from build123d import *

# Parameters (mm, degrees)
BOSS_EXTRUDE1_DEPTH                            = 76.2
CUT_EXTRUDE1_DEPTH                             = 15.24
CUT_EXTRUDE2_DEPTH                             = 15.24
CSK_FOR_M3_FLAT_HEAD_MACHINE_SCREW1_AT_2_COUNT = 2
CSK_FOR_M3_FLAT_HEAD_MACHINE_SCREW1_AT_2_PITCH = 59.436
CSK_FOR_M3_FLAT_HEAD_MACHINE_SCREW1_AT_3_COUNT = 2
CSK_FOR_M3_FLAT_HEAD_MACHINE_SCREW1_AT_3_PITCH = 29.851441177
M3_5_CLEARANCE_HOLE1_D                         = 3.96875
M3_5_CLEARANCE_HOLE1_DEPTH                     = 15.24
M3_5_CLEARANCE_HOLE2_D                         = 3.96875
M3_5_CLEARANCE_HOLE2_DEPTH                     = 15.24
M3_5_CLEARANCE_HOLE3_D                         = 3.96875
M3_5_CLEARANCE_HOLE3_DEPTH                     = 45.72
SKETCH21_R                                     = 2.5
CUT_EXTRUDE3_DEPTH                             = 1.5748


with BuildPart() as part:
    # Sketch1 → Boss-Extrude1 (new body)
    with BuildSketch(Plane.XY.offset(38.1)):
        with BuildLine():
            Line((25.4, -2.950829012), (25.4, -1.376029012))
            Line((25.4, -1.376029012), (3.278975474, -1.376029012))
            ThreePointArc((3.278975474, -1.376029012), (-2.746946179, 2.258190135), (1.984375, -2.950829012))
            Line((1.984375, -2.950829012), (25.4, -2.950829012))
        make_face()
    extrude(amount=-BOSS_EXTRUDE1_DEPTH)

    # Sketch6 → Cut-Extrude1 (cut)
    with BuildSketch(Plane(origin=(0, 0, -22.86), x_dir=(-1, 0, 0), z_dir=(0, 0, -1))):
        with BuildLine():
            Line((-3.937, -1.376029012), (-3.937, -2.950829012))
            Line((-3.937, -2.950829012), (-1.984375, -2.950829012))
            ThreePointArc((-1.984375, -2.950829012), (2.746946179, 2.258190135), (-3.278975474, -1.376029012))
            Line((-3.278975474, -1.376029012), (-3.937, -1.376029012))
        make_face()
    extrude(amount=-CUT_EXTRUDE1_DEPTH, mode=Mode.SUBTRACT)

    # Sketch12 → Cut-Extrude2 (cut)
    with BuildSketch(Plane(origin=(0, 0, 7.62), x_dir=(-1, 0, 0), z_dir=(0, 0, -1))):
        with BuildLine():
            Line((-3.937, -1.376029012), (-3.937, -2.950829012))
            Line((-3.937, -2.950829012), (-1.984375, -2.950829012))
            ThreePointArc((-1.984375, -2.950829012), (2.746946179, 2.258190135), (-3.278975474, -1.376029012))
            Line((-3.278975474, -1.376029012), (-3.937, -1.376029012))
        make_face()
    extrude(amount=-CUT_EXTRUDE2_DEPTH, mode=Mode.SUBTRACT)

    # Sketch13 → CSK for M3 Flat Head Machine Screw1 (revolve, cut)
    with BuildSketch(Plane(origin=(16.637, -1.376029012, -29.718), x_dir=(0, 0, 1), z_dir=(1, 0, 0))):
        Polygon((0, 0), (0, 2.179970988), (1.7526, 2.179970988), (1.7526, 0.7874), (2.437076377, 0), align=None)
    csk_for_m3_flat_head_machine_screw1 = revolve(axis=Axis((16.637, 4.973970988, -29.718), (0, -1, 0)), mode=Mode.SUBTRACT)

    # CSK for M3 Flat Head Machine Screw1 at 2: CSK for M3 Flat Head Machine Screw1 ×2
    with Locations(*[(0, 0, i * CSK_FOR_M3_FLAT_HEAD_MACHINE_SCREW1_AT_2_PITCH) for i in range(1, CSK_FOR_M3_FLAT_HEAD_MACHINE_SCREW1_AT_2_COUNT)]):
        add(csk_for_m3_flat_head_machine_screw1, mode=Mode.SUBTRACT)

    # CSK for M3 Flat Head Machine Screw1 at 3: CSK for M3 Flat Head Machine Screw1 ×2
    with Locations(*[Vector(0.094447701, 0, 0.995529825) * (i * CSK_FOR_M3_FLAT_HEAD_MACHINE_SCREW1_AT_3_PITCH) for i in range(1, CSK_FOR_M3_FLAT_HEAD_MACHINE_SCREW1_AT_3_COUNT)]):
        add(csk_for_m3_flat_head_machine_screw1, mode=Mode.SUBTRACT)

    # M3.5 Clearance Hole1
    with Locations(Plane.XY.offset(38.1)):
        with Locations((0, 0)):
            Hole(M3_5_CLEARANCE_HOLE1_D / 2, depth=M3_5_CLEARANCE_HOLE1_DEPTH)

    # M3.5 Clearance Hole2
    with Locations(Plane(origin=(0, 0, -38.1), x_dir=(-1, 0, 0), z_dir=(0, 0, -1))):
        with Locations((0, 0)):
            Hole(M3_5_CLEARANCE_HOLE2_D / 2, depth=M3_5_CLEARANCE_HOLE2_DEPTH)

    # M3.5 Clearance Hole3
    with Locations(Plane(origin=(0, 0, -7.62), x_dir=(-1, 0, 0), z_dir=(0, 0, -1))):
        with Locations((0, 0)):
            Hole(M3_5_CLEARANCE_HOLE3_D / 2, depth=M3_5_CLEARANCE_HOLE3_DEPTH)

    # Sketch21 → Cut-Extrude3 (cut)
    with BuildSketch(Plane(origin=(0, -1.376029012, 0), x_dir=(1, 0, 0), z_dir=(0, 1, 0))):
        with Locations((16.637, 29.718)):
            Circle(SKETCH21_R)
        with Locations((19.4564, 0)):
            Circle(SKETCH21_R)
        with Locations((16.637, -29.718)):
            Circle(SKETCH21_R)
    extrude(amount=-CUT_EXTRUDE3_DEPTH, mode=Mode.SUBTRACT)


solid = part.part
Source: CAD feature listing. Evaluate the final solid. Frame: model axes, mm. A direction names the side the tool comes from. Coordinates: 2 decimals unless noted, no trailing zeros. Loops run counter-clockwise (first coordinate to the right, second up) from the corner with the lowest first, then second, coordinate; pieces in that order, holes last. Notation, with made-up numbers: (4, 54.25) - (51, 54.25) arc R30 ccw to (51, 92.25) - close; hole circle Ø3 at (5, 65). An arc over 180 degrees is marked (long way). One line per item, written item: value. Start each with the question number.
1. Ray query, L1, parallel to Z at x = 1.75, y = 1; L2, parallel to Y at x = 0, z = 31.75; L3, parallel to Z at x = 18.5, y = -2.25. Return the intervals inside material, ascending.
2. Contact query for flat-ended pins moving along their axis: P1, Ø1.3, axis at y = -2, z = -19, coming from the -X side; P2, Ø3, axis at x = 17, z = 22.5, coming from the +Y side; P3, Ø11.5, axis at x = 14.5, z = 3, coming from the -Y side. Output: stop coordinate, or through.
3. Section A-A (z = 0). Return the cut outline in (x, y).
4. Set-up query: faces 1 (the flat face through (3.937, -2, -15)), 2 (the cylindrical face through (14.65, -2.15, -28.2)). Return all of +Z, -Z, +X, -X, +Y, -Y with unobstructed straight access to the full face (end or side cutting, diameter ignored); none if empty.
5. Section B-B (x = 0). Return the cut outline in (y, z), and give its area (3 significant figures).
6. Section D-D (x = 15). Return the cut outline in (y, z).
7. Mould query, pull axis X, two halves, no side actions, for faces 3 (the flat face through (25.4, -2, 1)), 4 (the cylindrical face through (14.653, -2.152, 31.239)), 5 (the flat face through (14, -2.951, 1)). Classes: pulls with the +X half, pulls with the -X half, needs draft (parallel to the pull), parting line crosses it, or undercut.
Verdict:
1. L1: z = -38.1 to -22.86, -7.62 to 7.62, 22.86 to 38.1
1. L2: y = -3.56 to -1.98, 1.98 to 3.56
1. L3: z = -38.1 to -31.39, -28.05 to -2.31, 2.31 to 28.05, 31.39 to 38.1
2. P1: stops at x = 3.94
2. P2: stops at y = -1.38
2. P3: stops at y = -2.95
3. outline: (1.98, -2.95) - (16.96, -2.95) - (16.96, -1.38) - (3.28, -1.38) arc R3.56 ccw (long way) to start; (21.96, -2.95) - (25.4, -2.95) - (25.4, -1.38) - (21.96, -1.38) - close; hole circle Ø3.97 at (0, 0)
4. face 1: -X, +Y, -Y
4. face 2: +Y, -Y
5. outline: (-3.56, -38.1) - (-1.98, -38.1) - (-1.98, -22.86) - (-3.56, -22.86) - close; (-3.56, -7.62) - (-1.98, -7.62) - (-1.98, 7.62) - (-3.56, 7.62) - close; (-3.56, 22.86) - (-1.98, 22.86) - (-1.98, 38.1) - (-3.56, 38.1) - close; (1.98, -38.1) - (3.56, -38.1) - (3.56, -22.86) - (1.98, -22.86) - close; (1.98, -7.62) - (3.56, -7.62) - (3.56, 7.62) - (1.98, 7.62) - close; (1.98, 22.86) - (3.56, 22.86) - (3.56, 38.1) - (1.98, 38.1) - close
5. area: 144 mm2
6. outline: (-2.95, -38.1) - (-1.38, -38.1) - (-1.38, -31.61) - (-2.95, -31.61) - close; (-2.95, -27.83) - (-1.38, -27.83) - (-1.38, 27.83) - (-2.95, 27.83) - close; (-2.95, 31.61) - (-1.38, 31.61) - (-1.38, 38.1) - (-2.95, 38.1) - close
7. face 3: pulls with the +X half
7. face 4: undercut
7. face 5: needs draft
